from build123d import *

# Parameters (mm, degrees)
SKETCH_W        = 120
SKETCH_H        = 135
PAD_DEPTH       = 3
POCKET_DEPTH    = 5
FILLET_R        = 5
SKETCH002_W     = 15
SKETCH002_H     = 30
POCKET001_DEPTH = 1
FILLET001_R     = 5


with BuildPart() as part:
    # Sketch → Pad (new body)
    with BuildSketch(Plane.XY):
        with Locations((60, 67.5)):
            Rectangle(SKETCH_W, SKETCH_H)
    extrude(amount=PAD_DEPTH)

    # Sketch001 → Pocket (cut)
    with BuildSketch(Plane.XY):
        with BuildLine():
            ThreePointArc((10, 22.5), (7.5, 25), (5, 22.5))
            Line((5, 22.5), (5, 7.5))
            ThreePointArc((5, 7.5), (7.5, 5), (10, 7.5))
            Line((10, 22.5), (10, 7.5))
        make_face()
        with BuildLine():
            ThreePointArc((115, 22.5), (112.5, 25), (110, 22.5))
            Line((110, 22.5), (110, 7.5))
            ThreePointArc((110, 7.5), (112.5, 5), (115, 7.5))
            Line((115, 22.5), (115, 7.5))
        make_face()
        with BuildLine():
            ThreePointArc((10, 127.5), (7.5, 130), (5, 127.5))
            Line((5, 127.5), (5, 112.5))
            ThreePointArc((5, 112.5), (7.5, 110), (10, 112.5))
            Line((10, 127.5), (10, 112.5))
        make_face()
        with BuildLine():
            ThreePointArc((115, 127.5), (112.5, 130), (110, 127.5))
            Line((110, 127.5), (110, 112.5))
            ThreePointArc((110, 112.5), (112.5, 110), (115, 112.5))
            Line((115, 127.5), (115, 112.5))
        make_face()
    extrude(amount=POCKET_DEPTH, mode=Mode.SUBTRACT)

    # Fillet
    fillet_edges = [part.edges().sort_by_distance(p)[0] for p in [
        (120, 0, 1.5),
        (120, 135, 1.5),
        (0, 135, 1.5),
        (0, 0, 1.5),
    ]]
    fillet(fillet_edges, radius=FILLET_R)

    # Sketch002 → Pocket001 (cut)
    with BuildSketch(Plane.XY):
        with Locations((7.5, 15)):
            Rectangle(SKETCH002_W, SKETCH002_H)
        with Locations((7.5, 120)):
            Rectangle(SKETCH002_W, SKETCH002_H)
        with Locations((112.5, 120)):
            Rectangle(SKETCH002_W, SKETCH002_H)
        with Locations((112.5, 15)):
            Rectangle(SKETCH002_W, SKETCH002_H)
    extrude(amount=POCKET001_DEPTH, mode=Mode.SUBTRACT)

    # Fillet001
    fillet001_edges = [part.edges().sort_by_distance(p)[0] for p in [
        (15, 105, 0.5),
        (105, 105, 0.5),
        (105, 30, 0.5),
        (15, 30, 0.5),
    ]]
    fillet(fillet001_edges, radius=FILLET001_R)


solid = part.part
CAD build for the part. Positions are in the model's coordinates, mm. A direction names the side the tool comes from. Round coordinates to 2 decimals unless told otherwise and drop trailing zeros. Order: outer loops, then holes, each group sorted by start corner. A loop starts at its lowest first (then second) coordinate and runs counter-clockwise, first axis right, second up. Notation, with made-up numbers: (-11, 3) -> (27, 3) arc R8 ccw to (27, 12) -> close; hole circle Ø2 at (18.25, 71.5). An arc over 180 degrees is marked (long way). Write each question's results on one line, items separated by ' | '.
1. Flat gauge pins, fed straight in: P1, Ø0.5, axis at y = 121.5, z = 0.5, coming from the +X side; P2, Ø12, axis at x = 115.5, y = 15.5, coming from the -Z side; P3, Ø0.5, axis at x = 2.5, z = 0.5, coming from the -Y side. Where does each tip first touch, or does it go through?
Findings below:
P1: stops at x = 105 | P2: stops at z = 1 | P3: stops at y = 30
2. Wall check: line 1 along X through (y, z) = (114.5, 2.15); line 2 along Y through (x, z) = (7, 2.4); line 3 along X through (y, z) = (112, 2.7). Give the ranges that are in metal, low to high. Write a range as [from, to].
Findings below:
line 1: x = [0, 5], [10, 110], [115, 120] | line 2: y = [0, 5.05], [24.95, 110.05], [129.95, 135] | line 3: x = [0, 5.05], [9.95, 110.05], [114.95, 120]
3. 3-axis set-ups, long thin cutter, end or side, ignore diameter. For faces 1 (the face through (4, 120, 1)), 2 (the face through (13.5, 28.57, 0.51)), 3 (the face through (106.43, 106.5, 0.51)), 4 (the face through (116, 15, 1)): which of +Z, -Z, +X, -X, +Y, -Y reach the whole face in a straight line?
Findings below:
face 1: -Z, -X, +Y | face 2: -Z, -X, -Y | face 3: -Z, +X, +Y | face 4: -Z, +X, -Y
4. Cut at B-B (x = 7.5). Give the cut face in (y, z).
Findings below:
outline: (0, 1) -> (5, 1) -> (5, 3) -> (0, 3) -> close; (25, 1) -> (30, 1) -> (30, 0) -> (105, 0) -> (105, 1) -> (110, 1) -> (110, 3) -> (25, 3) -> close; (130, 1) -> (135, 1) -> (135, 3) -> (130, 3) -> close
5. Cut at A-A (z = 2.15). Give the cut face in (x, y), plus the area to 3 significant figures.
Findings below:
outline: (0, 5) arc R5 ccw to (5, 0) -> (115, 0) arc R5 ccw to (120, 5) -> (120, 130) arc R5 ccw to (115, 135) -> (5, 135) arc R5 ccw to (0, 130) -> close; hole (5, 7.5) arc R2.5 ccw to (10, 7.5) -> (10, 22.5) arc R2.5 ccw to (5, 22.5) -> close; hole (5, 112.5) arc R2.5 ccw to (10, 112.5) -> (10, 127.5) arc R2.5 ccw to (5, 127.5) -> close; hole (110, 7.5) arc R2.5 ccw to (115, 7.5) -> (115, 22.5) arc R2.5 ccw to (110, 22.5) -> close; hole (110, 112.5) arc R2.5 ccw to (115, 112.5) -> (115, 127.5) arc R2.5 ccw to (110, 127.5) -> close | area: 15,800 mm²
6. Cut at C-C (x = 113). Give the cut face in (y, z), plus the area to 3 significant figures.
Findings below:
outline: (0, 1) -> (5.05, 1) -> (5.05, 3) -> (0, 3) -> close; (24.95, 1) -> (30, 1) -> (30, 0) -> (105, 0) -> (105, 1) -> (110.05, 1) -> (110.05, 3) -> (24.95, 3) -> close; (129.95, 1) -> (135, 1) -> (135, 3) -> (129.95, 3) -> close | area: 265 mm²
